Can you work these out from the model? Positions are in its coordinate system, mm. A direction names the side the tool comes from. Give positions to 0.01 mm unless a question says otherwise; leave off trailing zeros. Loops run counter-clockwise (first coordinate to the right, second up) from the corner with the lowest first, then second, coordinate; pieces in that order, holes last. Notation, with made-up numbers: (65.5, 5.25) - (116.5, 5.25) arc R31 cw to (116.5, 40.25) - close; hole circle Ø1 at (-31.5, 11.25). An arc over 180 degrees is marked (long way). Use a Markdown table: item, result. Add a question column.
```python
from build123d import *

# Parameters (mm, degrees)
SKETCH1_W           = 138
SKETCH1_H           = 83
SKETCH1_W_2         = 128
SKETCH1_H_2         = 73
BOSS_EXTRUDE1_DEPTH = 10
SKETCH2_W           = 5
SKETCH2_H           = 5
BOSS_EXTRUDE2_DEPTH = 5
SKETCH3_W           = 138
SKETCH3_H           = 5
BOSS_EXTRUDE3_DEPTH = 38
SKETCH6_W           = 138
SKETCH6_H           = 28
BOSS_EXTRUDE4_DEPTH = 5
BOSS_EXTRUDE5_DEPTH = 138
BOSS_EXTRUDE6_DEPTH = 5
BOSS_EXTRUDE7_DEPTH = 5
CUT_EXTRUDE1_REACH  = 97.915
SKETCH14_W          = 51
SKETCH14_H          = 20
SKETCH16_W          = 15
SKETCH16_H          = 13
CUT_EXTRUDE2_DEPTH  = 2
CUT_EXTRUDE3_REACH  = 96.631
SKETCH17_W          = 3
SKETCH17_H          = 13
SKETCH18_R          = 1
CUT_EXTRUDE4_DEPTH  = 3.5
CUT_EXTRUDE5_REACH  = 98.396
SKETCH19_R          = 2
SKETCH20_W          = 15
SKETCH20_H          = 4
CUT_EXTRUDE6_DEPTH  = 3


with BuildPart() as part:
    # Sketch1 → Boss-Extrude1 (new body)
    with BuildSketch(Plane.XY):
        Rectangle(SKETCH1_W, SKETCH1_H)
        Rectangle(SKETCH1_W_2, SKETCH1_H_2, mode=Mode.SUBTRACT)
    extrude(amount=BOSS_EXTRUDE1_DEPTH)

    # Sketch2 → Boss-Extrude2 (add)
    with BuildSketch(Plane.XY.offset(10)):
        with Locations((66.5, 39)):
            Rectangle(SKETCH2_W, SKETCH2_H)
        with Locations((66.5, -39)):
            Rectangle(SKETCH2_W, SKETCH2_H)
        with Locations((-66.5, -39)):
            Rectangle(SKETCH2_W, SKETCH2_H)
        with Locations((-66.5, 39)):
            Rectangle(SKETCH2_W, SKETCH2_H)
    extrude(amount=BOSS_EXTRUDE2_DEPTH)

    # Sketch3 → Boss-Extrude3 (add)
    with BuildSketch(Plane(origin=(0, 0, 0), x_dir=(-1, 0, 0), z_dir=(0, 0, -1))):
        with Locations((0, -39)):
            Rectangle(SKETCH3_W, SKETCH3_H)
    extrude(amount=BOSS_EXTRUDE3_DEPTH)

    # Sketch6 → Boss-Extrude4 (add)
    with BuildSketch(Plane.XY.offset(-38)):
        with Locations((0, -22.5)):
            Rectangle(SKETCH6_W, SKETCH6_H)
    extrude(amount=BOSS_EXTRUDE4_DEPTH)

    # Sketch8 → Boss-Extrude5 (add, through all)
    with BuildSketch(Plane(origin=(69, 0, 0), x_dir=(0, 0, -1), z_dir=(1, 0, 0))):
        Polygon((0, 41.5), (38, -8.5), (33, -8.5), (-5, 41.5), align=None)
    extrude(amount=-BOSS_EXTRUDE5_DEPTH)

    # Sketch9 → Boss-Extrude6 (add)
    with BuildSketch(Plane(origin=(69, 0, 0), x_dir=(0, 0, -1), z_dir=(1, 0, 0))):
        Polygon((0, 34.921052632), (33, -8.5), (33, -36.5), (0, -36.5), align=None)
    extrude(amount=-BOSS_EXTRUDE6_DEPTH)

    # Sketch10 → Boss-Extrude7 (add)
    with BuildSketch(Plane.ZY.offset(69)):
        Polygon((0, 34.921052632), (0, -36.5), (-33, -36.5), (-33, -8.5), align=None)
    extrude(amount=-BOSS_EXTRUDE7_DEPTH)

    # Sketch14 → Cut-Extrude1 (cut, up to next)
    with BuildSketch(Plane(origin=(0, 15.194219067, -19.992393509), x_dir=(-1, 0, 0), z_dir=(0, 0.6050832675335605, -0.7961621941231005)), mode=Mode.PRIVATE) as cut_extrude1_sk1:
        with Locations((-26.994700685, 1.64009412)):
            Rectangle(SKETCH14_W, SKETCH14_H)
    cut_extrude1_tool1 = extrude(cut_extrude1_sk1.sketch, amount=-CUT_EXTRUDE1_REACH, mode=Mode.PRIVATE) & part.part
    add(cut_extrude1_tool1.solids().sort_by_distance((26.994701, 16.5, -19))[0], mode=Mode.SUBTRACT)

    # Sketch16 → Cut-Extrude2 (cut)
    with BuildSketch(Plane(origin=(0, 15.194219067, -19.992393509), x_dir=(-1, 0, 0), z_dir=(0, 0.6050832675335606, -0.7961621941231006))):
        with Locations((46.5, 1.64009412)):
            Rectangle(SKETCH16_W, SKETCH16_H)
    extrude(amount=-CUT_EXTRUDE2_DEPTH, mode=Mode.SUBTRACT)

    # Sketch17 → Cut-Extrude3 (cut, up to next)
    with BuildSketch(Plane(origin=(0, 13.984052532, -18.400069121), x_dir=(-1, 0, 0), z_dir=(0, 0.6050832675335606, -0.7961621941231006)), mode=Mode.PRIVATE) as cut_extrude3_sk1:
        with Locations((40.5, 1.64009412)):
            Rectangle(SKETCH17_W, SKETCH17_H)
    cut_extrude3_tool1 = extrude(cut_extrude3_sk1.sketch, amount=-CUT_EXTRUDE3_REACH, mode=Mode.PRIVATE) & part.part
    # Sketch17 → Cut-Extrude3 (cut, up to next)
    with BuildSketch(Plane(origin=(0, 13.984052532, -18.400069121), x_dir=(-1, 0, 0), z_dir=(0, 0.6050832675335606, -0.7961621941231006)), mode=Mode.PRIVATE) as cut_extrude3_sk2:
        with Locations((52.5, 1.64009412)):
            Rectangle(SKETCH17_W, SKETCH17_H)
    cut_extrude3_tool2 = extrude(cut_extrude3_sk2.sketch, amount=-CUT_EXTRUDE3_REACH, mode=Mode.PRIVATE) & part.part
    add(cut_extrude3_tool1.solids().sort_by_distance((-40.5, 15.289833, -17.407676))[0], mode=Mode.SUBTRACT)
    add(cut_extrude3_tool2.solids().sort_by_distance((-52.5, 15.289833, -17.407676))[0], mode=Mode.SUBTRACT)

    # Sketch18 → Cut-Extrude4 (cut)
    with BuildSketch(Plane(origin=(0, 12.785496957, -16.823022312), x_dir=(1, 0, 0), z_dir=(0, -0.6050832675335605, 0.7961621941231007))):
        with Locations(Location((49.194700685, -10.13990588, 0), (0, 0, 270))):
            Circle(SKETCH18_R)
        with Locations(Location((4.794700685, -10.13990588, 0), (0, 0, 270))):
            Circle(SKETCH18_R)
        with Locations(Location((4.794700685, 13.42009412, 0), (0, 0, 270))):
            Circle(SKETCH18_R)
        with Locations(Location((49.194700685, 13.42009412, 0), (0, 0, 270))):
            Circle(SKETCH18_R)
    extrude(amount=-CUT_EXTRUDE4_DEPTH, mode=Mode.SUBTRACT)

    # Sketch19 → Cut-Extrude5 (cut, up to next)
    with BuildSketch(Plane(origin=(0, 0, -38), x_dir=(-1, 0, 0), z_dir=(0, 0, -1)), mode=Mode.PRIVATE) as cut_extrude5_sk1:
        with Locations((40, -25)):
            Circle(SKETCH19_R)
    cut_extrude5_tool1 = extrude(cut_extrude5_sk1.sketch, amount=-CUT_EXTRUDE5_REACH, mode=Mode.PRIVATE) & part.part
    # Sketch19 → Cut-Extrude5 (cut, up to next)
    with BuildSketch(Plane(origin=(0, 0, -38), x_dir=(-1, 0, 0), z_dir=(0, 0, -1)), mode=Mode.PRIVATE) as cut_extrude5_sk2:
        with Locations((0, -25)):
            Circle(SKETCH19_R)
    cut_extrude5_tool2 = extrude(cut_extrude5_sk2.sketch, amount=-CUT_EXTRUDE5_REACH, mode=Mode.PRIVATE) & part.part
    # Sketch19 → Cut-Extrude5 (cut, up to next)
    with BuildSketch(Plane(origin=(0, 0, -38), x_dir=(-1, 0, 0), z_dir=(0, 0, -1)), mode=Mode.PRIVATE) as cut_extrude5_sk3:
        with Locations((-40, -25)):
            Circle(SKETCH19_R)
    cut_extrude5_tool3 = extrude(cut_extrude5_sk3.sketch, amount=-CUT_EXTRUDE5_REACH, mode=Mode.PRIVATE) & part.part
    add(cut_extrude5_tool1.solids().sort_by_distance((-40, -25, -38))[0], mode=Mode.SUBTRACT)
    add(cut_extrude5_tool2.solids().sort_by_distance((0, -25, -38))[0], mode=Mode.SUBTRACT)
    add(cut_extrude5_tool3.solids().sort_by_distance((40, -25, -38))[0], mode=Mode.SUBTRACT)

    # Sketch20 → Cut-Extrude6 (cut)
    with BuildSketch(Plane(origin=(0, 12.785496957, -16.823022312), x_dir=(1, 0, 0), z_dir=(0, -0.6050832675335605, 0.7961621941231007))):
        with Locations((26.994700685, -10.35990588)):
            Rectangle(SKETCH20_W, SKETCH20_H)
    extrude(amount=-CUT_EXTRUDE6_DEPTH, mode=Mode.SUBTRACT)


solid = part.part
```
1. Suppose I cut it at B-B (z = 6). List the corners of the cut face in (x, y) for me, and give its area (3 significant figures).
2. Suppose I cut it at A-A (x = 40). List the corners of the cut face in (y, z) for me, and give its area (3 significant figures).
3. Suppose I cut it at C-C (y = -25). List the corners of the cut face in (x, z) for me.
4. If we mould it in two halves opening along X, with no side actions, what happens to faces 1 (the face through (34.495, 5, -24)), 2 (the face through (-69, -9, -11)), 3 (the face through (0.966, 16.85, -18.734))? For each: released by +X, released by -X, zero draft, split by the parting line, or undercut.
5. Will these pins go through, and if not, where does the flat tip stop? P1, Ø5.5, axis at x = 66.5, y = -9.5, coming from the +Z side; P2, Ø21.5, axis at x = 1.5, z = -5, coming from the +Y side; P3, Ø5, axis at x = 0, y = -25, coming from the +Z side; P4, Ø2, axis at x = -30.5, y = -5.5, coming from the -Z side.
6. On a 3-axis mill with a long thin cutter (end or side, diameter ignored), from which of +Z, -Z, +X, -X, +Y, -Y can I reach the whole of each face in a straight line? I mean faces 4 (the face through (-46.4, 20.76, -13.86)), 5 (the face through (66, -36.5, 12)), 6 (the face through (1, -36.5, -11)), 7 (the face through (-64, 39, 12)). Say none if no direction works.
7. Please list where these lines run through material, in increasing order: line 1 along X through (y, z) = (-12.5, -8); line 2 along Y through (x, z) = (-51, 2.5); line 3 along Z through (x, y) = (-29, -33.5). Write a range as [from, to].
8. Suppose I cut it at D-D (x = 0). List the corners of the cut face in (y, z) for me.
Results below:
| question | item | result |
|---|---|---|
| 1 | outline | (-69, -41.5) - (69, -41.5) - (69, 41.5) - (-69, 41.5) - close; hole (-64, -36.5) - (64, -36.5) - (64, 36.5) - (-64, 36.5) - close |
| 1 | area | 2,110 mm² |
| 2 | outline | (-41.5, -38) - (-27, -38) - (-27, -33) - (-36.5, -33) - (-36.5, 10) - (-41.5, 10) - close; (-23, -38) - (-8.5, -38) - (8.54, -25.05) - (6.13, -21.88) - (-8.5, -33) - (-23, -33) - close; (22.05, -9.78) - (24.46, -12.95) - (41.5, 0) - (41.5, 10) - (36.5, 10) - (36.5, 1.2) - close |
| 2 | area | 565 mm² |
| 3 | outline | (-69, -38) - (-42, -38) - (-42, -33) - (-64, -33) - (-64, 10) - (-69, 10) - close; (-38, -38) - (-2, -38) - (-2, -33) - (-38, -33) - close; (2, -38) - (38, -38) - (38, -33) - (2, -33) - close; (42, -38) - (69, -38) - (69, 10) - (64, 10) - (64, -33) - (42, -33) - close |
| 4 | face 1 | undercut |
| 4 | face 2 | released by -X |
| 4 | face 3 | zero draft |
| 5 | P1 | z = 10 |
| 5 | P2 | y = 41.5 |
| 5 | P3 | z = -33 |
| 5 | P4 | z = -36.48 |
| 6 | face 4 | -Z |
| 6 | face 5 | +Z, +X, -X |
| 6 | face 6 | +Z |
| 6 | face 7 | +Z, +Y, -Y |
| 7 | line 1 | [-69, -64], [64, 69] |
| 7 | line 2 | [-41.5, -36.5], [36.5, 41.5] |
| 7 | line 3 | [-38, -33] |
| 8 | outline | (-41.5, -38) - (-27, -38) - (-27, -33) - (-36.5, -33) - (-36.5, 10) - (-41.5, 10) - close; (-23, -38) - (-8.5, -38) - (41.5, 0) - (41.5, 10) - (36.5, 10) - (36.5, 1.2) - (-8.5, -33) - (-23, -33) - close |
